from build123d import *

# Parameters (mm, degrees)
SKETCH_1_W          = 140
SKETCH_1_H          = 140
EXTRUDE_1_DEPTH     = 2
SKETCH_2_R          = 2.525
CUT_EXTRUDE_1_DEPTH = 12
SKETCH_3_R          = 2.525
CUT_EXTRUDE_2_DEPTH = 17
SKETCH_4_OUTSIDE_W  = 181.606
SKETCH_4_OUTSIDE_H  = 181.606
CUT_EXTRUDE_3_DEPTH = 22
FILLET_1_R          = 3
FILLET_2_R          = 3
FILLET_3_R          = 5


with BuildPart() as part:
    # 草图1 → 凸台-拉伸1 (new, symmetric)
    with BuildSketch(Plane.XY):
        Rectangle(SKETCH_1_W, SKETCH_1_H)
    extrude(amount=EXTRUDE_1_DEPTH, both=True)

    # 草图2 → 切除-拉伸1 (cut, symmetric)
    with BuildSketch(Plane.XY.offset(2)):
        with Locations(Location((64, -64, 0), (0, 0, 180))):
            Circle(SKETCH_2_R)
    extrude(amount=CUT_EXTRUDE_1_DEPTH, both=True, mode=Mode.SUBTRACT)

    # 草图3 → 切除-拉伸2 (cut, symmetric)
    with BuildSketch(Plane.XY.offset(2)):
        with Locations(Location((63.551189893, 13.073625474, 0), (0, 0, 180))):
            Circle(SKETCH_3_R)
        with Locations(Location((22.804744615, 55.6226511, 0), (0, 0, 180))):
            Circle(SKETCH_3_R)
        with Locations(Location((-63.213858355, 55.65002484, 0), (0, 0, 180))):
            Circle(SKETCH_3_R)
    extrude(amount=CUT_EXTRUDE_2_DEPTH, both=True, mode=Mode.SUBTRACT)

    # 草图4 outside → 切除-拉伸3 (cut, symmetric)
    with BuildSketch(Plane(origin=(0, 0, -2), x_dir=(-1, 0, 0), z_dir=(0, 0, -1))):
        Rectangle(SKETCH_4_OUTSIDE_W, SKETCH_4_OUTSIDE_H)
        Polygon((-58, -70), (-58, 10.195392206), (-20.216854418, 49.65002484), (70, 49.65002484), (70, 61.6226511), (-25.366420755, 61.6226511), (-70, 15.014528745), (-70, -70), align=None, mode=Mode.SUBTRACT)
    extrude(amount=CUT_EXTRUDE_3_DEPTH, both=True, mode=Mode.SUBTRACT)

    # 圆角1
    fillet_1_edges = [part.edges().sort_by_distance(p)[0] for p in [
        (58, -70, 0),
        (70, -70, 0),
    ]]
    fillet(fillet_1_edges, radius=FILLET_1_R)

    # 圆角2
    fillet_2_edges = [part.edges().sort_by_distance(p)[0] for p in [
        (-70, 61.6226511, 0),
        (-70, 49.65002484, 0),
    ]]
    fillet(fillet_2_edges, radius=FILLET_2_R)

    # 圆角3
    fillet_3_edges = [part.edges().sort_by_distance(p)[0] for p in [
        (70, 15.014528745, 0),
        (25.366420755, 61.6226511, 0),
        (20.216854418, 49.65002484, 0),
        (58, 10.195392206, 0),
    ]]
    fillet(fillet_3_edges, radius=FILLET_3_R)


solid = part.part
Work out the finished part from the listing and answer in its coordinate system (mm). A direction names the side the tool comes from. Round coordinates to 2 decimals unless told otherwise and drop trailing zeros. Order: outer loops, then holes, each group sorted by start corner. A loop starts at its lowest first (then second) coordinate and runs counter-clockwise, first axis right, second up. Notation, with made-up numbers: M -3.5,28.25 L 34.5,28.25 A35 ccw 34.5,64.25 Z; hole C 63.5,86 d10. An arc over 180 degrees is marked long. Put each result on its own line as item: value. Start each with the question number.
Q1. Section C-C, the plane z = 0.45 is taken. Write down the section's boundary in (x, y) (3 decimals).
Q2. For a pull along X with two mould halves and no side action, classify faces 3 (the cylindrical face through (66.074, 12.963, 0.028)), 4 (the flat face through (39.4, 29.62, -0.03)), 5 (the flat face through (47.435, 38.578, -0.028)) as pulls with the +X half, pulls with the -X half, needs draft (parallel to the pull), parting line crosses it, or undercut.
Q3. Section B-B, the plane x = 64 is taken. Write down the section's boundary in (y, z) (3 decimals).
Q4. Straight lines are drawn through the part: L1, parallel to Y at x = 64, z = -0.5 (3 decimals); L2, parallel to Y at x = -59.5, z = -0.2; L3, parallel to X at y = -36.5, z = -1.45. For each, find the intervals that lie inside material, in ascending order. Write a range as [from, to].
Q5. Flat-ended cylindrical pins translate along their axes: pin 1 (2 mm diameter, centred on x = -24.5, z = 1, fed in from -Y); pin 2 (4.5 mm diameter, centred on x = 22.8, y = 55.62, fed in from +Z). Find the tip coordinate at first contact, or state that the pin passes through.
Q6. Section D-D, the plane y = -46 is taken. Write down the section's boundary in (x, z).
Q7. A tool of negligible diameter and unlimited length cuts with its end or side. For faces 1 (the flat face through (-70, 56, 0)), 2 (the flat face through (58, -30, 0)), from which of +Z, -Z, +X, -X, +Y, -Y can it reach the whole face along a straight path? Write none if from no direction.
Q8. Section A-A, the plane y = -64 is taken. Write down the section's boundary in (x, z) (3 decimals), and give its area (3 significant figures).
Findings below:
1. outline: M -70,52.65 A3 ccw -67,49.65 L 18.082,49.65 A5 cw 21.693,48.108 L 56.611,11.646 A5 cw 58,8.187 L 58,-67 A3 ccw 61,-70 L 67,-70 A3 ccw 70,-67 L 70,13.007 A5 ccw 68.611,16.465 L 26.843,60.081 A5 ccw 23.232,61.623 L -67,61.623 A3 ccw -70,58.623 Z; hole C -63.214,55.65 d5.05; hole C 22.805,55.623 d5.05; hole C 63.551,13.074 d5.05; hole C 64,-64 d5.05
2. face 3: undercut
2. face 4: pulls with the -X half
2. face 5: pulls with the +X half
3. outline: M -70,-2 L -66.525,-2 L -66.525,2 L -70,2 Z; M -61.475,-2 L 10.589,-2 L 10.589,2 L -61.475,2 Z; M 15.558,-2 L 21.28,-2 L 21.28,2 L 15.558,2 Z
4. L1: y = [-70, -66.525], [-61.475, 10.589], [15.558, 21.28]
4. L2: y = [49.65, 61.62]
4. L3: x = [58, 70]
5. pin 1: stops at y = 49.65
5. pin 2: passes through
6. outline: M 58,-2 L 70,-2 L 70,2 L 58,2 Z
7. face 1: +Z, -Z, -X, +Y, -Y
7. face 2: +Z, -Z, -X, -Y
8. outline: M 58,-2 L 61.475,-2 L 61.475,2 L 58,2 Z; M 66.525,-2 L 70,-2 L 70,2 L 66.525,2 Z
8. area: 27.8 mm^2
